CAD build for the part. Positions are in the model's coordinates, mm. A direction names the side the tool comes from. Give positions to 0.01 mm unless a question says otherwise; leave off trailing zeros. Write each loop counter-clockwise with the first axis right and the second up, starting at its lowest first coordinate (ties: lowest second). Pieces come first, ordered by that corner, then holes. Notation, with made-up numbers: (37, 69) -> (63, 69) arc R21 cw to (63, 97) -> close; hole circle Ø1 at (33, 75.25). An arc over 180 degrees is marked (long way). Answer as a JSON object with one key per item and string values.
```python
from build123d import *

# Parameters (mm, degrees)
SKETCH1_W           = 6.6
SKETCH1_H           = 20
BOSS_EXTRUDE1_DEPTH = 94.25
SKETCH3_W           = 10
SKETCH3_H           = 88.17
BOSS_EXTRUDE2_DEPTH = 6
SKETCH4_W           = 4.5
SKETCH4_H           = 85
BOSS_EXTRUDE3_DEPTH = 7.5


with BuildPart() as part:
    # Sketch1 → Boss-Extrude1 (new body)
    with BuildSketch(Plane(origin=(0, 0, 0), x_dir=(1, 0, 0), z_dir=(0, 1, 0))):
        with Locations((3.3, 10)):
            Rectangle(SKETCH1_W, SKETCH1_H)
    extrude(amount=BOSS_EXTRUDE1_DEPTH)

    # Sketch3 → Boss-Extrude2 (add)
    with BuildSketch(Plane.ZY):
        with Locations((-5, 50.165)):
            Rectangle(SKETCH3_W, SKETCH3_H)
    extrude(amount=BOSS_EXTRUDE2_DEPTH)

    # Sketch4 → Boss-Extrude3 (add)
    with BuildSketch(Plane(origin=(6.6, 0, 0), x_dir=(0, 0, -1), z_dir=(1, 0, 0))):
        with Locations((2.25, 51.75)):
            Rectangle(SKETCH4_W, SKETCH4_H)
    extrude(amount=BOSS_EXTRUDE3_DEPTH)


solid = part.part
```
1) Mould opens along X. For faces 1 (the flat face through (-6, 51, -5)), 2 (the flat face through (-3, 50, -10)), 3 (the flat face through (14.1, 52, -2)) say: released by +X, released by -X, zero draft, split by the parting line, or undercut.
Model answer:
{"face 1": "released by -X", "face 2": "zero draft", "face 3": "released by +X"}
2) Pin check, flat tips, straight feed: pin 1 (3 mm diameter, centred on x = -2, z = -5.5, fed in from -Y); pin 2 (2 mm diameter, centred on x = 9.5, y = 44, fed in from -Z); pin 3 (2 mm diameter, centred on y = 53, z = -16.5, fed in from +X). Stop position of each tip, or through.
Model answer:
{"pin 1": "stops at y = 6.08", "pin 2": "stops at z = -4.5", "pin 3": "stops at x = 6.6"}
3) 3-axis set-ups, long thin cutter, end or side, ignore diameter. For faces 4 (the flat face through (10, 9.25, -2)), 5 (the flat face through (10, 51, -4.5)), 6 (the flat face through (-3, 6.08, -5)): which of +Z, -Z, +X, -X, +Y, -Y reach the whole face in a straight line?
Model answer:
{"face 4": "+Z, -Z, +X, -Y", "face 5": "-Z, +X, +Y, -Y", "face 6": "+Z, -Z, -X, -Y"}
4) Slice it at B-B (y = 41.5). List the corners of the cut face in (x, z), then the cut area to 3 significant figures.
Model answer:
{"outline": "(-6, -10) -> (0, -10) -> (0, -20) -> (6.6, -20) -> (6.6, -4.5) -> (14.1, -4.5) -> (14.1, 0) -> (-6, 0) -> close", "area": "226 mm2"}
5) Slice it at D-D (z = -8). List the corners of the cut face in (x, y).
Model answer:
{"outline": "(-6, 6.08) -> (0, 6.08) -> (0, 0) -> (6.6, 0) -> (6.6, 94.25) -> (-6, 94.25) -> close"}
6) Wall check: probe 1 along Z at (x, y) = (11.5, 86.5); probe 2 along Z at (x, y) = (-1.5, 84); probe 3 along X at (y, z) = (48, -9.25). Give the ranges that are in metal, low to high.
Model answer:
{"probe 1": "z = -4.5 to 0", "probe 2": "z = -10 to 0", "probe 3": "x = -6 to 6.6"}
7) Slice it at C-C (x = 12). List the corners of the cut face in (y, z).
Model answer:
{"outline": "(9.25, -4.5) -> (94.25, -4.5) -> (94.25, 0) -> (9.25, 0) -> close"}
8) Slice it at A-A (z = -1.5). List the corners of the cut face in (x, y).
Model answer:
{"outline": "(-6, 6.08) -> (0, 6.08) -> (0, 0) -> (6.6, 0) -> (6.6, 9.25) -> (14.1, 9.25) -> (14.1, 94.25) -> (-6, 94.25) -> close"}
